The drawing under review shows one solid part. Ordinate dimensions are in mm from its lowest x, y, z. A direction names the side the tool comes from. Round coordinates to 2 decimals unless told otherwise and drop trailing zeros. Write each loop counter-clockwise with the first axis right and the second up, starting at its lowest first coordinate (ties: lowest second). Pieces come first, ordered by that corner, then holes. Notation, with made-up numbers: (29.5, 35) -> (74.5, 35) arc R10 cw to (74.5, 53) -> close; hole circle Ø11 at (4.25, 67). An arc over 180 degrees is marked (long way). Write item = value, one per line. Start each with the question number.
Item 1: Add section B-B, the plane y = 5.75. State the section outline as (x, z) points (1 decimal).
Item 2: Add section A-A, the plane x = 6.5. State the section outline as (y, z) points.
Item 3: Machinability: for the marked faces 3 and 4, which of the approach directions +Z, -Z, +X, -X, +Y, -Y give a long, thin tool a straight path to every point of the face, cutting with its end or side? Answer none if there is none.
Item 4: To check wall thickness, follow L1, parallel to Y at x = 6.5, z = 9.25; L2, parallel to Y at x = 6.5, z = 2.9. State the ranges of each line that lie inside material, in increasing order.
Item 5: Mouldability with a two-part tool opening along Y and no side actions: class the marked faces 1 and 2 as released by +Y, released by -Y, zero draft, split by the parting line, or undercut.
Item 6: Add section C-C, the plane z = 5.75. State the section outline as (x, y) points.
Item 7: Add section D-D, the plane y = 2.5. State the section outline as (x, z) points, then the cut area to 3 significant figures.
Item 8: For pin 1 Ø5 at (y, z) = (11, 12) entering from +X (1 decimal); pin 2 Ø2 at (x, z) = (1.5, 2) entering from -Y; pin 3 Ø7.5 at (x, y) = (6.5, 6.5) entering from +Z, all flat-tipped, find the tip position at first contact; note any pin that passes through.
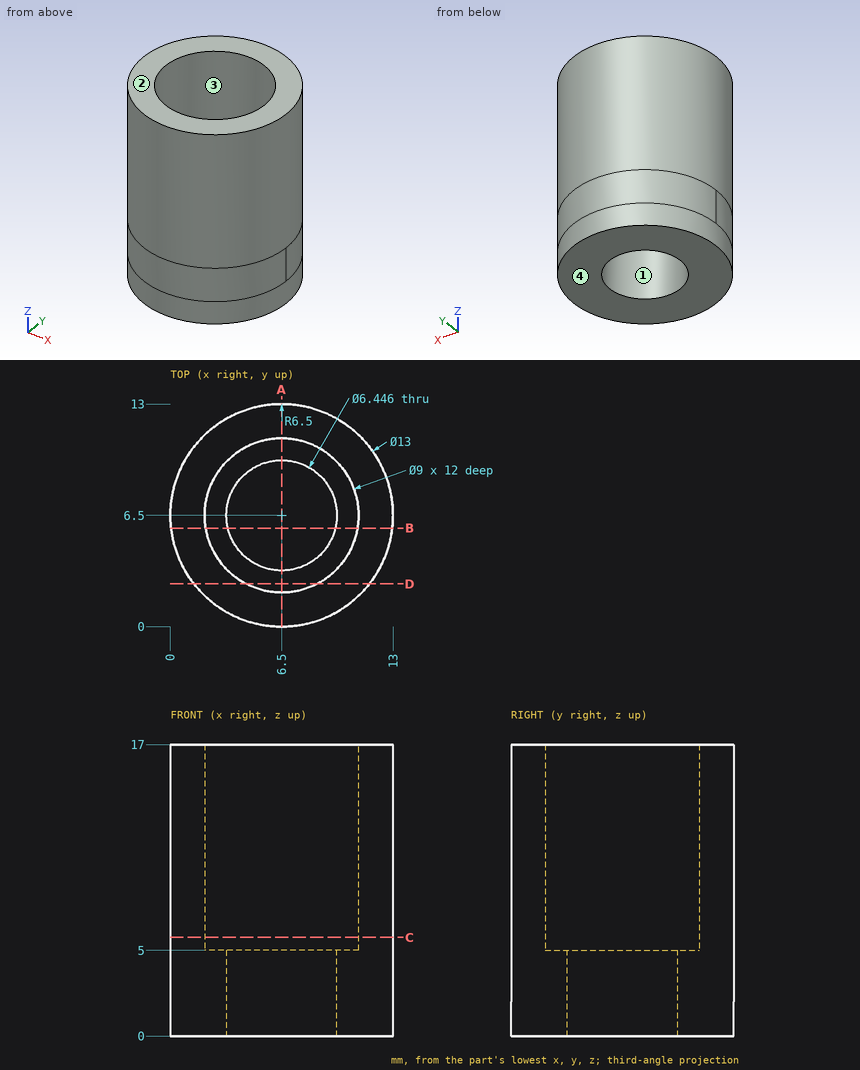
Result set:
q1.outline = (0, 0) -> (3.4, 0) -> (3.4, 5) -> (2.1, 5) -> (2.1, 17) -> (0, 17) -> close; (9.6, 0) -> (13, 0) -> (13, 17) -> (10.9, 17) -> (10.9, 5) -> (9.6, 5) -> close
q2.outline = (0, 0) -> (3.28, 0) -> (3.28, 5) -> (2, 5) -> (2, 17) -> (0, 17) -> close; (9.72, 0) -> (13, 0) -> (13, 17) -> (11, 17) -> (11, 5) -> (9.72, 5) -> close
q3.face_3 = +Z
q3.face_4 = -Z, +X, -X, +Y, -Y
q4.L1 = 0 to 2, 11 to 13
q4.L2 = 0 to 3.28, 9.72 to 13
q5.face_1 = undercut
q5.face_2 = zero draft
q6.outline = circle Ø13 at (6.5, 6.5); hole circle Ø9 at (6.5, 6.5)
q7.outline = (1.38, 0) -> (11.62, 0) -> (11.62, 17) -> (8.56, 17) -> (8.56, 5) -> (4.44, 5) -> (4.44, 17) -> (1.38, 17) -> close
q7.area = 125 mm²
q8.pin_1 = 12.7
q8.pin_2 = 1.38
q8.pin_3 = 5
